```python
from build123d import *

# Parameters (mm, degrees)
SKETCH3_W                = 25.5
SKETCH3_H                = 15.5
BOSS_EXTRUDE2_DEPTH      = 18
SKETCH4_W                = 22.6
SKETCH4_H                = 12.6
CUT_EXTRUDE1_DEPTH       = 15
SKETCH7_W                = 25.5
SKETCH7_H                = 3
BOSS_EXTRUDE4_DEPTH      = 10
BOSS_EXTRUDE4_DEPTH_BACK = 25.5
SKETCH8_R                = 1.98
CUT_EXTRUDE2_DEPTH       = 16
CUT_EXTRUDE2_DEPTH_BACK  = 31
BOSS_EXTRUDE5_DEPTH      = 25.5
SKETCH10_W               = 15
SKETCH10_H               = 7.75
CUT_EXTRUDE3_DEPTH       = 5
CUT_EXTRUDE3_DEPTH_BACK  = 9


with BuildPart() as part:
    # Sketch3 → Boss-Extrude2 (new body)
    with BuildSketch(Plane.XY):
        with Locations((12.75, 7.75)):
            Rectangle(SKETCH3_W, SKETCH3_H)
    extrude(amount=BOSS_EXTRUDE2_DEPTH)

    # Sketch4 → Cut-Extrude1 (cut)
    with BuildSketch(Plane.XY.offset(18)):
        with Locations((12.750003743, 7.749991635)):
            Rectangle(SKETCH4_W, SKETCH4_H)
    extrude(amount=-CUT_EXTRUDE1_DEPTH, mode=Mode.SUBTRACT)

    # Sketch7 → Boss-Extrude4 (add, two sides)
    with BuildSketch(Plane.XZ) as boss_extrude4_sk:
        with Locations((12.75, 1.5)):
            Rectangle(SKETCH7_W, SKETCH7_H)
    extrude(amount=BOSS_EXTRUDE4_DEPTH)
    extrude(boss_extrude4_sk.sketch, amount=-BOSS_EXTRUDE4_DEPTH_BACK)

    # Sketch8 → Cut-Extrude2 (cut, two sides)
    with BuildSketch(Plane.XY.offset(3)) as cut_extrude2_sk:
        with Locations((19.125, 20.5)):
            Circle(SKETCH8_R)
        with Locations((6.375, -5)):
            Circle(SKETCH8_R)
        with Locations((6.375, 20.5)):
            Circle(SKETCH8_R)
        with Locations((19.125, -5)):
            Circle(SKETCH8_R)
    extrude(amount=CUT_EXTRUDE2_DEPTH, mode=Mode.SUBTRACT)
    extrude(cut_extrude2_sk.sketch, amount=-CUT_EXTRUDE2_DEPTH_BACK, mode=Mode.SUBTRACT)

    # Sketch9 → Boss-Extrude5 (add)
    with BuildSketch(Plane.ZY):
        Polygon((3, 17.01), (3, 15.5), (4.51, 15.5), align=None)
        Polygon((4.51, 0), (3, 0), (3, -1.51), align=None)
    extrude(amount=-BOSS_EXTRUDE5_DEPTH)

    # Sketch10 → Cut-Extrude3 (cut, two sides)
    with BuildSketch(Plane(origin=(25.5, 0, 0), x_dir=(0, 0, -1), z_dir=(1, 0, 0))) as cut_extrude3_sk:
        with Locations((-10.5, 7.75)):
            Rectangle(SKETCH10_W, SKETCH10_H)
    extrude(amount=CUT_EXTRUDE3_DEPTH, mode=Mode.SUBTRACT)
    extrude(cut_extrude3_sk.sketch, amount=-CUT_EXTRUDE3_DEPTH_BACK, mode=Mode.SUBTRACT)


solid = part.part
```
The listing builds one solid part. Answer for the finished solid, in the listing's coordinates (mm). A direction names the side the tool comes from. Give positions to 0.01 mm unless a question says otherwise; leave off trailing zeros. Loops run counter-clockwise (first coordinate to the right, second up) from the corner with the lowest first, then second, coordinate; pieces in that order, holes last. Notation, with made-up numbers: M -32.5,28 L -17.5,28 A12 cw -17.5,49 Z; hole C 43,-18 d4. An arc over 180 degrees is marked long. One line per item, written item: value.
1. Each of these flat-tipped pins is pushed along its axis until it touches: P1, Ø4.5, axis at x = 18, z = 12, coming from the +Y side; P2, Ø5, axis at x = 9.5, z = 8, coming from the -Y side; P3, Ø7, axis at x = 13.5, y = 21.5, coming from the +Z side. Where does it stop, or does it pass through?
Found:
P1: y = 15.5
P2: y = 0
P3: z = 3
2. Section B-B on y = 20 is taken. Determine the outline of the cut face in (x, z), plus the area to 3 significant figures.
Found:
outline: M 0,0 L 4.46,0 L 4.46,3 L 0,3 Z; M 8.29,0 L 17.21,0 L 17.21,3 L 8.29,3 Z; M 21.04,0 L 25.5,0 L 25.5,3 L 21.04,3 Z
area: 53.5 mm^2
3. For faces 1 (the face through (13, -6, 3)), 2 (the face through (24.05, 3, 11)), 3 (the face through (25, 3.875, 11)), determine the directions among +Z, -Z, +X, -X, +Y, -Y from which every point of the face is accessible in a straight line to the end or side of a thin tool.
Found:
face 1: +Z, +X, -X, -Y
face 2: +Z
face 3: +Z, +X
4. Section D-D on y = -5 is taken. Determine the outline of the cut face in (x, z) (3 decimals), plus the area to 3 significant figures.
Found:
outline: M 0,0 L 4.395,0 L 4.395,3 L 0,3 Z; M 8.355,0 L 17.145,0 L 17.145,3 L 8.355,3 Z; M 21.105,0 L 25.5,0 L 25.5,3 L 21.105,3 Z
area: 52.7 mm^2
5. Find the intervals of material crossed by probe 1 along Y at (x, z) = (8.25, 7); probe 2 along X at (y, z) = (1.5, 15.25); probe 3 along Z at (x, y) = (7.75, 8), in increasing order.
Found:
probe 1: 0 to 1.45, 14.05 to 15.5
probe 2: 0 to 1.45, 24.05 to 25.5
probe 3: 0 to 3
6. For a pull along Y with two mould halves and no side action, classify faces 4 (the face through (13, 8, 0)), 5 (the face through (13, 25.5, 2)), 6 (the face through (25, 11.625, 11)) as pulls with the +Y half, pulls with the -Y half, needs draft (parallel to the pull), parting line crosses it, or undercut.
Found:
face 4: needs draft
face 5: pulls with the +Y half
face 6: undercut
7. Section C-C on z = 8.5 is taken. Determine the outline of the cut face in (x, y) (3 decimals).
Found:
outline: M 0,0 L 25.5,0 L 25.5,3.875 L 24.05,3.875 L 24.05,1.45 L 1.45,1.45 L 1.45,14.05 L 24.05,14.05 L 24.05,11.625 L 25.5,11.625 L 25.5,15.5 L 0,15.5 Z
8. Section A-A on x = 19.75 is taken. Determine the outline of the cut face in (y, z).
Found:
outline: M -10,0 L -6.88,0 L -6.88,3 L -10,3 Z; M -3.12,0 L 18.62,0 L 18.62,3 L 17.01,3 L 15.5,4.51 L 15.5,18 L 14.05,18 L 14.05,3 L 1.45,3 L 1.45,18 L 0,18 L 0,4.51 L -1.51,3 L -3.12,3 Z; M 22.38,0 L 25.5,0 L 25.5,3 L 22.38,3 Z
